The model under review builds one solid part; all positions refer to its coordinate system, in mm. A direction names the side the tool comes from. Round coordinates to 2 decimals unless told otherwise and drop trailing zeros. Order: outer loops, then holes, each group sorted by start corner. A loop starts at its lowest first (then second) coordinate and runs counter-clockwise, first axis right, second up. Notation, with made-up numbers: M -9.75,-31.75 L 47.25,-31.75 A25 ccw 47.25,5.25 Z; hole C -3,3 d11. An arc over 180 degrees is marked long. Use a Markdown table: item, result. Add a question column.
1. Consider section C-C on y = 25.5. State the section outline as (x, z) points.
2. Consider section B-B on z = 2.65. State the section outline as (x, y) points.
3. Consider section D-D on x = 0. State the section outline as (y, z) points, then the cut area to 3 significant figures.
4. The part is to be moulded in two halves that separate along Y. For faces 1 (the flat face through (5.4, 32.4, 4)), 2 (the cylindrical face through (-10.3, 37, 2)), 3 (the cylindrical face through (-11, 62.57, 1.97)), say which applies: +Y half, -Y half, draft (parallel to the pull), parting line (faces both ways), or undercut.
5. For faces 4 (the cylindrical face through (0.1, 7.5, 2)), 5 (the flat face through (0, 64, 2)), list the 3-axis set-ups (+Z, -Z, +X, -X, +Y, -Y) from which the entire face can be reached by the end or side of a thin tool; tool diameter is ignored.
6. To check wall thickness, follow probe 1 along X at (y, z) = (18, 1.45); probe 2 along X at (y, z) = (44.5, 2); probe 3 along Y at (x, z) = (-10.5, 0.95). State the ranges of each line that lie inside material, in increasing order.
7. Consider section A-A on y = 46. State the section outline as (x, z) points.
from build123d import *

# Parameters (mm, degrees)
DODANIE_WYCI_GNI_CIE1_DEPTH = 4


with BuildPart() as part:
    # Szkic1 → Dodanie-wyciągnięcie1 (new body)
    with BuildSketch(Plane.XY):
        with BuildLine():
            Line((-12.5, 0), (12.5, 0))
            Line((12.5, 0), (12.5, 59))
            ThreePointArc((12.5, 59), (11.035533906, 62.535533906), (7.5, 64))
            Line((7.5, 64), (-7.5, 64))
            ThreePointArc((-7.5, 64), (-11.035533906, 62.535533906), (-12.5, 59))
            Line((-12.5, 59), (-12.5, 0))
        make_face()
        with BuildLine():
            Line((5, 54), (5, 12.5))
            ThreePointArc((5, 12.5), (0, 7.5), (-5, 12.5))
            Line((-5, 12.5), (-5, 54))
            ThreePointArc((-5, 54), (0, 59), (5, 54))
        make_face(mode=Mode.SUBTRACT)
        with BuildLine():
            Line((-9, 35.75), (-9, 12.25))
            ThreePointArc((-9, 12.25), (-10.25, 11), (-11.5, 12.25))
            Line((-11.5, 12.25), (-11.5, 35.75))
            ThreePointArc((-11.5, 35.75), (-10.25, 37), (-9, 35.75))
        make_face(mode=Mode.SUBTRACT)
        with BuildLine():
            Line((9, 35.75), (9, 12.25))
            ThreePointArc((9, 12.25), (10.25, 11), (11.5, 12.25))
            Line((11.5, 12.25), (11.5, 35.75))
            ThreePointArc((11.5, 35.75), (10.25, 37), (9, 35.75))
        make_face(mode=Mode.SUBTRACT)
    extrude(amount=DODANIE_WYCI_GNI_CIE1_DEPTH)


solid = part.part
Answer block:
| question | item | result |
|---|---|---|
| 1 | outline | M -12.5,0 L -11.5,0 L -11.5,4 L -12.5,4 Z; M -9,0 L -5,0 L -5,4 L -9,4 Z; M 5,0 L 9,0 L 9,4 L 5,4 Z; M 11.5,0 L 12.5,0 L 12.5,4 L 11.5,4 Z |
| 2 | outline | M -12.5,0 L 12.5,0 L 12.5,59 A5 ccw 7.5,64 L -7.5,64 A5 ccw -12.5,59 Z; hole M -11.5,12.25 A1.25 ccw -9,12.25 L -9,35.75 A1.25 ccw -11.5,35.75 Z; hole M -5,12.5 A5 ccw 5,12.5 L 5,54 A5 ccw -5,54 Z; hole M 9,12.25 A1.25 ccw 11.5,12.25 L 11.5,35.75 A1.25 ccw 9,35.75 Z |
| 3 | outline | M 0,0 L 7.5,0 L 7.5,4 L 0,4 Z; M 59,0 L 64,0 L 64,4 L 59,4 Z |
| 3 | area | 50.0 mm^2 |
| 4 | face 1 | draft |
| 4 | face 2 | undercut |
| 4 | face 3 | +Y half |
| 5 | face 4 | +Z, -Z |
| 5 | face 5 | +Z, -Z, +X, -X, +Y |
| 6 | probe 1 | -12.5 to -11.5, -9 to -5, 5 to 9, 11.5 to 12.5 |
| 6 | probe 2 | -12.5 to -5, 5 to 12.5 |
| 6 | probe 3 | 0 to 11.03, 36.97 to 63 |
| 7 | outline | M -12.5,0 L -5,0 L -5,4 L -12.5,4 Z; M 5,0 L 12.5,0 L 12.5,4 L 5,4 Z |
